from build123d import *

# Parameters (mm, degrees)
F1_DEPTH = 3.96875


with BuildPart() as f1:
    # F0 (on Top) → F1 (new body)
    with BuildSketch(Plane.XY):
        with BuildLine():
            Line((6.357343, 3.599845), (6.327746, 3.651619))
            ThreePointArc((6.327746, 3.651619), (3.176014, 4.937132), (-0.214079, 4.631808))
            ThreePointArc((-0.214079, 4.631808), (-3.435517, 4.94244), (-6.411583, 3.670753))
            ThreePointArc((-6.411583, 3.670753), (-5.947905, 0.406573), (-4.103787, -2.326392))
            ThreePointArc((-4.103787, -2.326392), (-2.598583, -5.259348), (-0.090588, -7.398935))
            ThreePointArc((-0.090588, -7.398935), (2.544544, -5.363511), (3.970517, -2.354611))
            ThreePointArc((3.970517, -2.354611), (5.704057, 0.406109), (6.357343, 3.599845))
        make_face()
    extrude(amount=F1_DEPTH)


solid = f1.part
Input: part model. Units: mm. Frame: model coordinates. Give positions to 0.01 mm unless a question says otherwise; leave off trailing zeros. Write each loop counter-clockwise with the first axis right and the second up, starting at its lowest first coordinate (ties: lowest second). Pieces come first, ordered by that corner, then holes. Notation, with made-up numbers: M 52,27.25 L 71,27.25 A21 ccw 71,31.25 Z; hole C 4,-4 d3. An arc over 180 degrees is marked long. Write item = value, one per line. Start each with the question number.
1) Cut plane A-A on z = 2.05. Return the cut outline in (x, y), then the cut area to 3 significant figures.
2) Cut plane B-B on y = -5.25. Return the cut outline in (x, z), then the cut area to 3 significant figures.
3) Cut plane C-C on x = -2. Return the cut outline in (y, z).
4) Material intervals for line 1 along X through (y, z) = (3, 3.7); line 2 along Y through (x, z) = (3, 3.2); line 3 along Y through (x, z) = (-1.75, 1.6), sorted ascending. Write a range as [from, to].
5) Draft query along X for faces 1 (the cylindrical face through (3.22, 4.93, 1.96)), 2 (the cylindrical face through (2.515, -5.4, 1.957)), 3 (the cylindrical face through (-2.63, -5.22, 1.96)), 4 (the flat face through (0, 0, 3.969)). Return one class per face: +X half, -X half, draft (parallel to the pull), parting line (faces both ways), or undercut.
6) First-contact query: pin 1 Ø2 at (y, z) = (2, 3) entering from +X. Flat tip, straight axial feed; report the tip coordinate or a pass-through.
Solved:
q1.outline = M -6.41,3.67 A7.35 ccw -4.1,-2.33 A8.5 ccw -0.09,-7.4 A7.14 ccw 3.97,-2.35 A9.13 ccw 6.36,3.6 L 6.33,3.65 A7.2 ccw -0.21,4.63 A6.54 ccw Z
q1.area = 108 mm2
q2.outline = M -2.61,0 L 2.63,0 L 2.63,3.97 L -2.61,3.97 Z
q2.area = 20.8 mm2
q3.outline = M -5.94,0 L 5.01,0 L 5.01,3.97 L -5.94,3.97 Z
q4.line_1 = [-6.44, 6.32]
q4.line_2 = [-4.73, 4.96]
q4.line_3 = [-6.18, 4.98]
q5.face_1 = undercut
q5.face_2 = +X half
q5.face_3 = -X half
q5.face_4 = draft
q6.pin_1 = 6.32
